Could you check a few things on this drawing? It's one solid part, dimensions in mm from its lowest x, y, z. A direction names the side the tool comes from. Coordinates: 2 decimals unless noted, no trailing zeros. Order: outer loops, then holes, each group sorted by start corner. A loop starts at its lowest first (then second) coordinate and runs counter-clockwise, first axis right, second up.
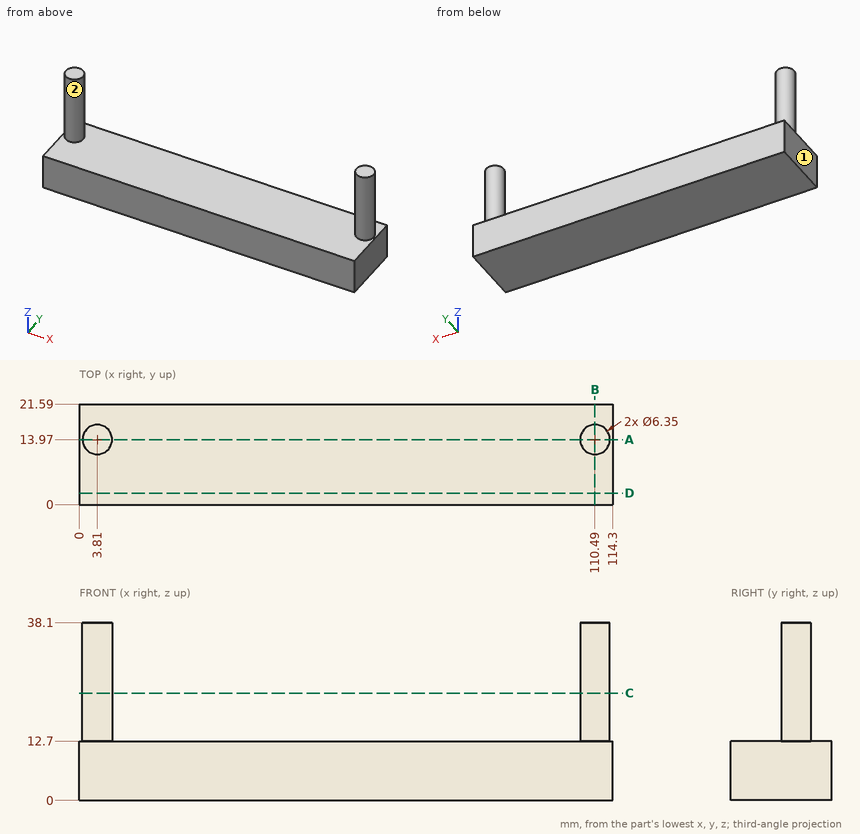
1. On a 3-axis mill with a long thin cutter (end or side, diameter ignored), from which of +Z, -Z, +X, -X, +Y, -Y can I reach the whole of each face in a straight line? I mean the marked faces 1 and 2. Say none if no direction works.
Completed:
face 1: +Z, -Z, -X, +Y, -Y
face 2: +Z
2. Imagine slicing it at B-B on x = 110.49. Please give me the cut outline in (y, z) (3 decimals), then the cut area to 3 significant figures.
Completed:
outline: (0, 0) - (21.59, 0) - (21.59, 12.7) - (17.145, 12.7) - (17.145, 38.1) - (10.795, 38.1) - (10.795, 12.7) - (0, 12.7) - close
area: 435 mm2
3. Imagine slicing it at C-C on z = 23. Please give me the cut outline in (x, y) (3 decimals), then the cut area to 3 significant figures.
Completed:
outline: circle Ø6.35 at (3.81, 13.97); circle Ø6.35 at (110.49, 13.97)
area: 63.3 mm2
4. Imagine slicing it at A-A on y = 13.97. Please give me the cut outline in (x, z) (3 decimals).
Completed:
outline: (0, 0) - (114.3, 0) - (114.3, 12.7) - (113.665, 12.7) - (113.665, 38.1) - (107.315, 38.1) - (107.315, 12.7) - (6.985, 12.7) - (6.985, 38.1) - (0.635, 38.1) - (0.635, 12.7) - (0, 12.7) - close
5. Imagine slicing it at D-D on y = 2.5. Please give me the cut outline in (x, z), then the cut area to 3 significant figures.
Completed:
outline: (0, 0) - (114.3, 0) - (114.3, 12.7) - (0, 12.7) - close
area: 1,450 mm2
6. I'm going to push flat-ended pins straight in: pin 1 (12 mm diameter, centred on x = 86, z = 16.5, fed in from +Y); pin 2 (10 mm diameter, centred on y = 14, z = 33, fed in from -X) (3 decimals); pin 3 (10 mm diameter, centred on y = 5, z = 32, fed in from +X); pin 4 (6.5 mm diameter, centred on x = 29, y = 5.5, fed in from +Z). Where does each tip first touch, or does it pass through?
Completed:
pin 1: stops at y = 21.59
pin 2: stops at x = 0.635
pin 3: passes through
pin 4: stops at z = 12.7
7. Please list where these lines run through material, in increasing order: probe 1 along Z at (x, y) = (22, 13.25); probe 2 along X at (y, z) = (11.25, 26); probe 3 along X at (y, z) = (11.5, 14.5).
Completed:
probe 1: z = 0 to 12.7
probe 2: x = 2.17 to 5.45, 108.85 to 112.13
probe 3: x = 1.82 to 5.8, 108.5 to 112.48
